Model file for the job. Use its own axes, mm. A direction names the side the tool comes from. Round coordinates to 2 decimals unless told otherwise and drop trailing zeros. Loops run counter-clockwise (first coordinate to the right, second up) from the corner with the lowest first, then second, coordinate; pieces in that order, holes last. Notation, with made-up numbers: (76, 14) -> (117, 14) arc R32 cw to (117, 50) -> close; hole circle Ø2 at (75, -29.75). An arc over 180 degrees is marked (long way). Use a Markdown table: item, result.
from build123d import *

# Parameters (mm, degrees)
SKETCH1_W               = 150
SKETCH1_H               = 55
BOSS_EXTRUDE1_DEPTH     = 2
SKETCH2_R               = 3.5
BOSS_EXTRUDE2_DEPTH     = 15
CUT_EXTRUDE1_REACH      = 83.672
SKETCH3_R               = 1.25
FILLET1_R               = 5
F_1_4_CLEARANCE_HOLE1_D = 7.14248
SKETCH8_R               = 2.1
CUT_EXTRUDE2_DEPTH      = 10


with BuildPart() as part:
    # Sketch1 → Boss-Extrude1 (new body)
    with BuildSketch(Plane(origin=(0, 0, 0), x_dir=(1, 0, 0), z_dir=(0, 1, 0))):
        Rectangle(SKETCH1_W, SKETCH1_H)
    extrude(amount=BOSS_EXTRUDE1_DEPTH)

    # Sketch2 → Boss-Extrude2 (add)
    with BuildSketch(Plane(origin=(0, 2, 0), x_dir=(1, 0, 0), z_dir=(0, 1, 0))):
        with Locations(Location((-67.75, -24, 0), (0, 0, 270))):
            Circle(SKETCH2_R)
        with Locations(Location((-67.75, 19.5, 0), (0, 0, 90))):
            Circle(SKETCH2_R)
        with Locations(Location((67.75, 19.5, 0), (0, 0, 90))):
            Circle(SKETCH2_R)
        with Locations(Location((67.75, -24, 0), (0, 0, 270))):
            Circle(SKETCH2_R)
    extrude(amount=BOSS_EXTRUDE2_DEPTH)

    # Sketch3 → Cut-Extrude1 (cut, up to next)
    with BuildSketch(Plane(origin=(0, 17, 0), x_dir=(1, 0, 0), z_dir=(0, 1, 0)), mode=Mode.PRIVATE) as cut_extrude1_sk1:
        with Locations(Location((-67.75, -24, 0), (0, 0, 270))):
            Circle(SKETCH3_R)
    cut_extrude1_tool1 = extrude(cut_extrude1_sk1.sketch, amount=-CUT_EXTRUDE1_REACH, mode=Mode.PRIVATE) & part.part
    # Sketch3 → Cut-Extrude1 (cut, up to next)
    with BuildSketch(Plane(origin=(0, 17, 0), x_dir=(1, 0, 0), z_dir=(0, 1, 0)), mode=Mode.PRIVATE) as cut_extrude1_sk2:
        with Locations(Location((-67.75, 19.5, 0), (0, 0, 270))):
            Circle(SKETCH3_R)
    cut_extrude1_tool2 = extrude(cut_extrude1_sk2.sketch, amount=-CUT_EXTRUDE1_REACH, mode=Mode.PRIVATE) & part.part
    # Sketch3 → Cut-Extrude1 (cut, up to next)
    with BuildSketch(Plane(origin=(0, 17, 0), x_dir=(1, 0, 0), z_dir=(0, 1, 0)), mode=Mode.PRIVATE) as cut_extrude1_sk3:
        with Locations(Location((67.75, 19.5, 0), (0, 0, 270))):
            Circle(SKETCH3_R)
    cut_extrude1_tool3 = extrude(cut_extrude1_sk3.sketch, amount=-CUT_EXTRUDE1_REACH, mode=Mode.PRIVATE) & part.part
    # Sketch3 → Cut-Extrude1 (cut, up to next)
    with BuildSketch(Plane(origin=(0, 17, 0), x_dir=(1, 0, 0), z_dir=(0, 1, 0)), mode=Mode.PRIVATE) as cut_extrude1_sk4:
        with Locations(Location((67.75, -24, 0), (0, 0, 270))):
            Circle(SKETCH3_R)
    cut_extrude1_tool4 = extrude(cut_extrude1_sk4.sketch, amount=-CUT_EXTRUDE1_REACH, mode=Mode.PRIVATE) & part.part
    add(cut_extrude1_tool1.solids().sort_by_distance((-67.75, 17, 24))[0], mode=Mode.SUBTRACT)
    add(cut_extrude1_tool2.solids().sort_by_distance((-67.75, 17, -19.5))[0], mode=Mode.SUBTRACT)
    add(cut_extrude1_tool3.solids().sort_by_distance((67.75, 17, -19.5))[0], mode=Mode.SUBTRACT)
    add(cut_extrude1_tool4.solids().sort_by_distance((67.75, 17, 24))[0], mode=Mode.SUBTRACT)

    # Fillet1
    fillet1_edges = [part.edges().sort_by_distance(p)[0] for p in [
        (75, 1, 27.5),
        (-75, 1, 27.5),
        (-75, 1, -27.5),
        (75, 1, -27.5),
    ]]
    fillet(fillet1_edges, radius=FILLET1_R)

    # 1/4 Clearance Hole1 (through all)
    with Locations(Plane(origin=(0, 2, 0), x_dir=(1, 0, 0), z_dir=(0, 1, 0))):
        with Locations((-50.8, 12.7), (50.8, 12.7), (50.8, -12.7), (-50.8, -12.7), (0, -12.7), (0, 12.7)):
            Hole(F_1_4_CLEARANCE_HOLE1_D / 2)

    # Sketch8 → Cut-Extrude2 (cut)
    with BuildSketch(Plane.XZ):
        with Locations(Location((-67.75, 24, 0), (0, 0, 270))):
            Circle(SKETCH8_R)
        with Locations(Location((-67.75, -19.5, 0), (0, 0, 270))):
            Circle(SKETCH8_R)
        with Locations(Location((67.75, -19.5, 0), (0, 0, 270))):
            Circle(SKETCH8_R)
        with Locations(Location((67.75, 24, 0), (0, 0, 270))):
            Circle(SKETCH8_R)
    extrude(amount=-CUT_EXTRUDE2_DEPTH, mode=Mode.SUBTRACT)


solid = part.part
Q1. Band-saw the part on D-D, the plane y = 13.5. Give the cut face in (x, z).
Results list:
| item | result |
|---|---|
| outline | circle Ø7 at (-67.75, -19.5); circle Ø7 at (-67.75, 24); circle Ø7 at (67.75, -19.5); circle Ø7 at (67.75, 24); hole circle Ø2.5 at (-67.75, -19.5); hole circle Ø2.5 at (-67.75, 24); hole circle Ø2.5 at (67.75, -19.5); hole circle Ø2.5 at (67.75, 24) |
Q2. Band-saw the part on C-C, the plane x = 50.8. Give the cut face in (y, z), plus the area to 3 significant figures.
Results list:
| item | result |
|---|---|
| outline | (0, -27.5) -> (2, -27.5) -> (2, -16.27) -> (0, -16.27) -> close; (0, -9.13) -> (2, -9.13) -> (2, 9.13) -> (0, 9.13) -> close; (0, 16.27) -> (2, 16.27) -> (2, 27.5) -> (0, 27.5) -> close |
| area | 81.4 mm² |
Q3. Band-saw the part on B-B, the plane z = 12.7. Give the cut face in (x, y).
Results list:
| item | result |
|---|---|
| outline | (-75, 0) -> (-54.37, 0) -> (-54.37, 2) -> (-75, 2) -> close; (-47.23, 0) -> (-3.57, 0) -> (-3.57, 2) -> (-47.23, 2) -> close; (3.57, 0) -> (47.23, 0) -> (47.23, 2) -> (3.57, 2) -> close; (54.37, 0) -> (75, 0) -> (75, 2) -> (54.37, 2) -> close |
Q4. Drill centre lines: L1, parallel to Z at x = -50.8, y = 1.6; L2, parallel to X at y = 1.35, z = -12.7; L3, parallel to X at y = 14.5, z = 24. Where is each one in solid material? Low to high. Write a range as from..to.
Results list:
| item | result |
|---|---|
| L1 | z = -27.5..-16.27, -9.13..9.13, 16.27..27.5 |
| L2 | x = -75..-54.37, -47.23..-3.57, 3.57..47.23, 54.37..75 |
| L3 | x = -71.25..-69, -66.5..-64.25, 64.25..66.5, 69..71.25 |
Q5. Band-saw the part on A-A, the plane y = 4.25. Give the cut face in (x, z).
Results list:
| item | result |
|---|---|
| outline | circle Ø7 at (-67.75, -19.5); circle Ø7 at (-67.75, 24); circle Ø7 at (67.75, -19.5); circle Ø7 at (67.75, 24); hole circle Ø4.2 at (-67.75, -19.5); hole circle Ø4.2 at (-67.75, 24); hole circle Ø4.2 at (67.75, -19.5); hole circle Ø4.2 at (67.75, 24) |
Q6. Tool access for faces 1 (the face through (-68, 10, -21)), 2 (the face through (-1, 2, 0)), 3 (the face through (73.5, 1.01, -26.07)): list every direction of +Z, -Z, +X, -X, +Y, -Y with a clear straight run to the whole face (end or side of a thin tool).
Results list:
| item | result |
|---|---|
| face 1 | -Y |
| face 2 | +Y |
| face 3 | -Z, +X, +Y, -Y |
Q7. Pull direction Z, two halves, no side cores. Call faces 4 (the face through (69.3, 17, -19.5)), 5 (the face through (-69, 10, 23)), 6 (the face through (73.5, 1.01, 26.07)): released by +Z, released by -Z, zero draft, split by the parting line, or undercut.
Results list:
| item | result |
|---|---|
| face 4 | zero draft |
| face 5 | undercut |
| face 6 | released by +Z |
Q8. Flat gauge pins, fed straight in: pin 1 (5.5 mm diameter, centred on x = -50.8, z = 12.7, fed in from -Y); pin 2 (3 mm diameter, centred on x = -58, z = 9, fed in from +Y); pin 3 (3.5 mm diameter, centred on x = -67.75, z = 24, fed in from -Y). Where does each tip first touch, or does it go through?
Results list:
| item | result |
|---|---|
| pin 1 | passes through |
| pin 2 | stops at y = 2 |
| pin 3 | stops at y = 10 |
